from build123d import *

# Parameters (mm, degrees)
EXTRUDE_1_DEPTH     = 7.6
CUT_EXTRUDE_1_DEPTH = 3.7
SKETCH_5_R          = 4.1
CUT_EXTRUDE_2_DEPTH = 3.7


with BuildPart() as part:
    # 草图1 → 凸台-拉伸1 (new, symmetric)
    with BuildSketch(Plane.XY):
        with BuildLine():
            Line((-7.348183963, -6.11049447), (-10.699512046, -7.67324442))
            ThreePointArc((-10.699512046, -7.67324442), (-12.619347786, -7.547411737), (-13.544748569, -5.860628846))
            Line((-13.544748569, -5.860628846), (-13.544748569, -2))
            ThreePointArc((-13.544748569, -2), (-12.958962131, -0.585786438), (-11.544748569, 0))
            Line((-11.544748569, 0), (11.255251431, 0))
            ThreePointArc((11.255251431, 0), (12.669464993, -0.585786438), (13.255251431, -2))
            Line((13.255251431, -2), (13.255251431, -5.860628846))
            ThreePointArc((13.255251431, -5.860628846), (12.329850648, -7.547411737), (10.410014907, -7.67324442))
            Line((10.410014907, -7.67324442), (7.058686825, -6.11049447))
            Line((7.058686825, -6.11049447), (7.481305087, -5.204186683))
            Line((7.481305087, -5.204186683), (10.832633169, -6.766936633))
            ThreePointArc((10.832633169, -6.766936633), (11.792551039, -6.704020292), (12.255251431, -5.860628846))
            Line((12.255251431, -5.860628846), (12.255251431, -2))
            ThreePointArc((12.255251431, -2), (11.962358212, -1.292893219), (11.255251431, -1))
            Line((11.255251431, -1), (-11.544748569, -1))
            ThreePointArc((-11.544748569, -1), (-12.25185535, -1.292893219), (-12.544748569, -2))
            Line((-12.544748569, -2), (-12.544748569, -5.860628846))
            ThreePointArc((-12.544748569, -5.860628846), (-12.082048177, -6.704020292), (-11.122130307, -6.766936633))
            Line((-11.122130307, -6.766936633), (-7.770802225, -5.204186683))
            Line((-7.770802225, -5.204186683), (-7.348183963, -6.11049447))
        make_face()
    extrude(amount=EXTRUDE_1_DEPTH, both=True)

    # 草图3 → 切除-拉伸1 (cut)
    with BuildSketch(Plane.XY.offset(7.6)):
        Polygon((-11.894748569, -3.292064446), (-5.65074495, -3.292064446), (-5.65074495, -8.789099245), (-21.304410353, -8.789099245), (-21.304410353, 0.944175246), (-11.894748569, 0.944175246), align=None)
        Polygon((5.361247812, -3.292064446), (5.361247812, -8.789099245), (21.014913215, -8.789099245), (21.014913215, 0.944175246), (11.605251431, 0.944175246), (11.605251431, -3.292064446), align=None)
    cut_extrude_1 = extrude(amount=-CUT_EXTRUDE_1_DEPTH, mode=Mode.SUBTRACT)

    # 镜向1: 切除-拉伸1 across plane
    add(cut_extrude_1.mirror(Plane.XY), mode=Mode.SUBTRACT)

    # 草图5 → 切除-拉伸2 (cut)
    with BuildSketch(Plane(origin=(0, 0, 0), x_dir=(1, 0, 0), z_dir=(0, 1, 0))):
        with Locations(Location((-0.144748569, 0, 0), (0, 0, 270))):
            Circle(SKETCH_5_R)
    extrude(amount=-CUT_EXTRUDE_2_DEPTH, mode=Mode.SUBTRACT)


solid = part.part
Work out the finished part from the listing and answer in its coordinate system (mm). A direction names the side the tool comes from. Give positions to 0.01 mm unless a question says otherwise; leave off trailing zeros. Write each loop counter-clockwise with the first axis right and the second up, starting at its lowest first coordinate (ties: lowest second). Pieces come first, ordered by that corner, then holes. Notation, with made-up numbers: (-38.75, -21.5) - (-4.75, -21.5) arc R24 ccw to (-4.75, -8.5) - close; hole circle Ø10 at (86.5, -34.75). An arc over 180 degrees is marked (long way). One line per item, written item: value. Start each with the question number.
1. For faces 4 (the flat face through (-11.895, -0.5, -5.8)), 5 (the flat face through (8.758, -6.903, 0.055)), 6 (the flat face through (12.255, -4, 0)), determine the directions among +Z, -Z, +X, -X, +Y, -Y from which every point of the face is accessible in a straight line to the end or side of a thin tool.
2. Find section D-D (z = -4.5). Write down the section's boundary in (x, y), then the cut area to 3 significant figures.
3. Given pin 1 (0.5 mm diameter, centred on y = -0.5, z = 6, fed in from -X); pin 2 (2 mm diameter, centred on x = 5.5, z = -1, fed in from +Y); pin 3 (7.5 mm diameter, centred on x = -3.5, z = -2, fed in from -Y); pin 4 (1.1 mm diameter, centred on y = -0.5, z = -5.5, fed in from +X), each flat-ended and moving along its own axis, determine where each tip first touches the part or whether it passes through.
4. Find section B-B (y = -3.25). Write down the section's boundary in (x, z).
5. Find section A-A (z = 0). Write down the section's boundary in (x, y), then the cut area to 3 significant figures.
6. For a pull along X with two mould halves and no side action, classify faces 1 (the flat face through (11.605, -0.5, -5.8)), 2 (the flat face through (-7.562, -5.651, 0.055)), 3 (the flat face through (0, -0.5, 7.6)) as +X half, -X half, draft (parallel to the pull), parting line (faces both ways), or undercut.
7. Find section C-C (x = 8). Write down the section's boundary in (y, z).
8. Consider probe 1 along X at (y, z) = (-5, -3.25); probe 2 along X at (y, z) = (-0.5, 0); probe 3 along Y at (x, z) = (-5, 6.5). Determine where each line is inside the solid, lowest interval first.
Geometry results:
1. face 4: -Z, -X, +Y, -Y
1. face 5: +Z, -Z, -Y
1. face 6: +Z, -Z
2. outline: (-11.89, -1.06) arc R1 cw to (-11.54, -1) - (11.26, -1) arc R1 cw to (11.61, -1.06) - (11.61, -0.03) arc R2 ccw to (11.26, 0) - (-11.54, 0) arc R2 ccw to (-11.89, -0.03) - close
2. area: 23.5 mm2
3. pin 1: x = -11.89
3. pin 2: y = 0
3. pin 3: y = -1
3. pin 4: x = 11.61
4. outline: (-13.54, -3.9) - (-12.54, -3.9) - (-12.54, 3.9) - (-13.54, 3.9) - close; (12.26, -3.9) - (13.26, -3.9) - (13.26, 3.9) - (12.26, 3.9) - close
5. outline: (-13.54, -5.86) arc R2 ccw to (-10.7, -7.67) - (-7.35, -6.11) - (-7.77, -5.2) - (-11.12, -6.77) arc R1 cw to (-12.54, -5.86) - (-12.54, -2) arc R1 cw to (-11.54, -1) - (-4.24, -1) - (-4.24, 0) - (-11.54, 0) arc R2 ccw to (-13.54, -2) - close; (3.96, -1) - (11.26, -1) arc R1 cw to (12.26, -2) - (12.26, -5.86) arc R1 cw to (10.83, -6.77) - (7.48, -5.2) - (7.06, -6.11) - (10.41, -7.67) arc R2 ccw to (13.26, -5.86) - (13.26, -2) arc R2 ccw to (11.26, 0) - (3.96, 0) - close
5. area: 40.5 mm2
6. face 1: +X half
6. face 2: undercut
6. face 3: draft
7. outline: (-6.55, -3.9) - (-5.45, -3.9) - (-5.45, 3.9) - (-6.55, 3.9) - close; (-1, -7.6) - (0, -7.6) - (0, 7.6) - (-1, 7.6) - close
8. probe 1: -13.54 to -12.54, 12.26 to 13.26
8. probe 2: -12.87 to -4.24, 3.96 to 12.58
8. probe 3: -1 to 0
